```python
from build123d import *

# Parameters (mm, degrees)
F0_R          = 4.7625
F1_DEPTH      = 152.4
F2_W          = 6.35
F2_H          = 4.7452268491
F5_DEPTH      = 4.7635
F5_DEPTH_BACK = 4.7635
F6_R          = 2.38125
F7_DEPTH      = 12.7


with BuildPart() as f1:
    # F0 (on Front) → F1 (new body)
    with BuildSketch(Plane.XZ):
        Circle(F0_R)
    extrude(amount=F1_DEPTH)

    # F2 (on Right) → F3 (revolve, cut)
    with BuildSketch(Plane.YZ):
        with Locations((-149.225, 4.7500534246)):
            Rectangle(F2_W, F2_H)
    revolve(axis=Axis((0, -25.3480933607, 0), (0, -1, 0)), mode=Mode.SUBTRACT)

    # F4 (on Right) → F5 (cut, two sides)
    with BuildSketch(Plane.YZ) as f5_sk:
        Polygon((0, -1.5875), (0, 0), (0, 1.5875), (-12.7, 1.5875), (-12.7, 0), (-12.7, -1.5875), align=None)
    extrude(amount=-F5_DEPTH, mode=Mode.SUBTRACT)
    extrude(f5_sk.sketch, amount=F5_DEPTH_BACK, mode=Mode.SUBTRACT)

    # F6 (on Top) → F7 (cut, symmetric)
    with BuildSketch(Plane.XY):
        with Locations((0, -3.81)):
            Circle(F6_R)
    extrude(amount=F7_DEPTH, both=True, mode=Mode.SUBTRACT)


solid = f1.part
```
Work out the finished part from the listing and answer in its coordinate system (mm). A direction names the side the tool comes from. Round coordinates to 2 decimals unless told otherwise and drop trailing zeros. Order: outer loops, then holes, each group sorted by start corner. A loop starts at its lowest first (then second) coordinate and runs counter-clockwise, first axis right, second up.
Q1. A cutting plane is placed at B-B, the plane y = -3.81. Determine the outline of the cut face in (x, z) (1 decimal), then the cut area to 3 significant figures.
Solution:
outline: (-4.5, -1.6) arc R4.8 ccw to (-2.4, -4.1) - (-2.4, -1.6) - close; (-4.5, 1.6) - (-2.4, 1.6) - (-2.4, 4.1) arc R4.8 ccw to start; (2.4, -4.1) arc R4.8 ccw to (4.5, -1.6) - (2.4, -1.6) - close; (2.4, 1.6) - (4.5, 1.6) arc R4.8 ccw to (2.4, 4.1) - close
area: 13.3 mm2
Q2. A tool of negligible diameter and unlimited length cuts with its end or side. For faces 4 (the flat face through (0, 0, -3)), 5 (the flat face through (0, -8, 1.588)), 6 (the flat face through (2, -146.05, -2)), from which of +Z, -Z, +X, -X, +Y, -Y can it reach the whole face along a straight path? Write none if from no direction.
Solution:
face 4: +Z, -Z, +X, -X, +Y
face 5: +X, -X, +Y
face 6: -Y
Q3. The mould has two halves that part along X. Classify faces 1 (the cylindrical face through (-1.03, -72, -4.65)), 2 (the cylindrical face through (-1.89, -5.26, 3.2)), 3 (the flat face through (0, -152.4, 0)): pulls with the +X half, pulls with the -X half, needs draft (parallel to the pull), parting line crosses it, or undercut.
Solution:
face 1: parting line crosses it
face 2: undercut
face 3: needs draft
Q4. A cutting plane is placed at D-D, the plane y = -121. Determine the outline of the cut face in (x, z) (1 decimal), then the cut area to 3 significant figures.
Solution:
outline: circle Ø9.5 at (0, 0)
area: 71.3 mm2
Q5. Given pin 1 Ø1 at (x, z) = (1, 0.5) entering from +Y; pin 2 Ø1.5 at (x, z) = (-3, 1) entering from -Y; pin 3 Ø1.5 at (y, z) = (-34, 3.5) entering from +X, each flat-ended and moving along its own axis, determine where each tip first touches the part or whether it passes through.
Solution:
pin 1: stops at y = -12.7
pin 2: stops at y = -146.05
pin 3: stops at x = 3.89
Q6. Find the intervals of material crossed by line 1 along Y through (x, z) = (0, -4.1); line 2 along X through (y, z) = (-101.5, -0.25); line 3 along Y through (x, z) = (-2.25, 0.25), in increasing order.
Solution:
line 1: y = -146.05 to -6.19, -1.43 to 0
line 2: x = -4.76 to 4.76
line 3: y = -152.4 to -12.7
Q7. A cutting plane is placed at C-C, the plane z = 0. Determine the outline of the cut face in (x, y).
Solution:
outline: (-4.76, -146.05) - (-2.38, -146.05) - (-2.38, -152.4) - (2.38, -152.4) - (2.38, -146.05) - (4.76, -146.05) - (4.76, -12.7) - (-4.76, -12.7) - close
Q8. A cutting plane is placed at A-A, the plane x = 0. Determine the outline of the cut face in (y, z), then the cut area to 3 significant figures.
Solution:
outline: (-152.4, -2.38) - (-146.05, -2.38) - (-146.05, -4.76) - (-6.19, -4.76) - (-6.19, -1.59) - (-12.7, -1.59) - (-12.7, 1.59) - (-6.19, 1.59) - (-6.19, 4.76) - (-146.05, 4.76) - (-146.05, 2.38) - (-152.4, 2.38) - close; (-1.43, -4.76) - (0, -4.76) - (0, -1.59) - (-1.43, -1.59) - close; (-1.43, 1.59) - (0, 1.59) - (0, 4.76) - (-1.43, 4.76) - close
area: 1,350 mm2
